from build123d import *

# Parameters (mm, degrees)
F0_W     = 150
F0_H     = 200
F0_R     = 5
F1_DEPTH = 25


with BuildPart() as f1:
    # F0 (on Front) → F1 (new body)
    with BuildSketch(Plane.XZ):
        with Locations((-25.85324, 64.885747)):
            Rectangle(F0_W, F0_H)
        with Locations((-87.344356, -29.108832)):
            Circle(F0_R, mode=Mode.SUBTRACT)
        with Locations((26.225695, 56.396399)):
            Circle(F0_R, mode=Mode.SUBTRACT)
        Polygon((49.14676, -35.114253), (-100.85324, -35.114253), (-158.585042, -58.980666), (-226.017654, -79.6455), (-254.655804, -135.114253), (45.344196, -135.114253), align=None)
    extrude(amount=F1_DEPTH)


solid = f1.part
The model under review builds one solid part; all positions refer to its coordinate system, in mm. A direction names the side the tool comes from. Round coordinates to 2 decimals unless told otherwise and drop trailing zeros. Write each loop counter-clockwise with the first axis right and the second up, starting at its lowest first coordinate (ties: lowest second). Pieces come first, ordered by that corner, then holes. Notation, with made-up numbers: (-28.5, 22) - (-16.5, 22) arc R26 ccw to (-16.5, 58) - close; hole circle Ø4 at (-1.5, -31.75). An arc over 180 degrees is marked (long way). One line per item, written item: value. Start each with the question number.
1. Consider section A-A on y = -13. Write out the cut boundary in (x, z), and give its area (3 significant figures).
2. Machinability: for faces 4 (the face through (49.147, -12, 63)), 5 (the face through (-100.853, -12, 63)), which of the approach directions +Z, -Z, +X, -X, +Y, -Y give a long, thin tool a straight path to every point of the face, cutting with its end or side? Answer none if there is none.
3. To check wall thickness, follow L1, parallel to Z at x = 26.5, y = -18.75; L2, parallel to X at y = -19, z = 90.5; L3, parallel to X at y = -14.5, z = -114.5. State the ranges of each line that lie inside material, in increasing order. Write a range as from..to.
4. Consider section C-C on x = -171.5. Write out the cut boundary in (y, z), and give its area (3 significant figures).
5. The part is to be moulded in two halves that separate along Z. For faces 1 (the face through (28.914, -12.325, 60.612)), 2 (the face through (-240.136, -12.325, -106.992)), 3 (the face through (47.22, -12.32, -85.81)), say which applies: released by +Z, released by -Z, zero draft, split by the parting line, or undercut.
6. Consider section B-B on z = 145. Write out the cut boundary in (x, y).
7. Clearance check with flat-ended pins moving along their axes: P1, Ø3, axis at x = -176.5, y = -3.5, coming from the +Z side; P2, Ø5, axis at y = -19, z = -20, coming from the -X side; P3, Ø1.5, axis at x = -159, y = -4, coming from the +Z side. State where each tip first meets the part, or that it passes through.
Checks:
1. outline: (-254.66, -135.11) - (45.34, -135.11) - (49.15, -35.11) - (49.15, 164.89) - (-100.85, 164.89) - (-100.85, -35.11) - (-158.59, -58.98) - (-226.02, -79.65) - close; hole circle Ø10 at (-87.34, -29.11); hole circle Ø10 at (26.23, 56.4)
1. area: 55,000 mm^2
2. face 4: +Z, -Z, +X, +Y, -Y
2. face 5: +Z, -X, +Y, -Y
3. L1: z = -135.11..51.4, 61.39..164.89
3. L2: x = -100.85..49.15
3. L3: x = -244.01..46.13
4. outline: (-25, -135.11) - (0, -135.11) - (0, -62.94) - (-25, -62.94) - close
4. area: 1,800 mm^2
5. face 1: undercut
5. face 2: released by +Z
5. face 3: released by -Z
6. outline: (-100.85, -25) - (49.15, -25) - (49.15, 0) - (-100.85, 0) - close
7. P1: stops at z = -64.01
7. P2: stops at x = -100.85
7. P3: stops at z = -58.84
